The listing builds one solid part. Answer for the finished solid, in the listing's coordinates (mm). A direction names the side the tool comes from. Coordinates: 2 decimals unless noted, no trailing zeros. Loops run counter-clockwise (first coordinate to the right, second up) from the corner with the lowest first, then second, coordinate; pieces in that order, holes last. Notation, with made-up numbers: M 73,-2.5 L 95,-2.5 A29 ccw 95,27.5 Z; hole C 42.5,25 d1. An arc over 180 degrees is marked long. Return JSON: item names as keys, results as strings. Group by question number.
1. Section C-C (x = 83.5) is taken. Write down the section's boundary in (y, z).
2. Which of the six approach directions +Z, -Z, +X, -X, +Y, -Y give full straight-line access (tool end or side, diameter ignored) to faces 4 (the face through (66.5, 0, -6)), 5 (the face through (8, -8, -8)), 6 (the face through (78.189, 10.382, -19.961)), 7 (the face through (19.8, -12.1, -9.2))?
3. Section A-A (x = 47.5) is taken. Write down the section's boundary in (y, z), then the cut area to 3 significant figures.
4. Section B-B (x = 13) is taken. Write down the section's boundary in (y, z).
5. The mould has two halves that part along Z. Classify faces 1 (the face through (94.5, 10, -11.5)), 2 (the face through (80.695, -11.521, -8.834)), 3 (the face through (35.099, -14.985, 0.66)): pulls with the +Z half, pulls with the -Z half, needs draft (parallel to the pull), parting line crosses it, or undercut.
6. Given P1, Ø3, axis at x = 57, y = 6.5, coming from the +Z side; P2, Ø3, axis at x = 60, y = -5, coming from the -Z side; P3, Ø10, axis at x = 50, z = 1, coming from the +Y side, each flat-ended and moving along its own axis, determine where each tip first touches the part or whether it passes through.
7. Straight lines are drawn through the part: L1, parallel to Z at x = 57, y = 0; L2, parallel to Y at x = 67, z = 5; L3, parallel to Z at x = 62.25, y = 0. For each, find the intervals that lie inside material, in ascending order. Write a range as from..to.
```python
from build123d import *


with BuildPart() as part:
    # Sketch1 → Revolve1 (revolve)
    with BuildSketch(Plane.XY):
        with BuildLine():
            Line((44.5, 5.1), (41.555513627, 0))
            Line((41.555513627, 0), (0, 0))
            Line((0, 0), (0, 10))
            Line((0, 10), (1, 11))
            Line((1, 11), (8, 11))
            Line((8, 11), (8, 19))
            Line((8, 19), (16, 19))
            Line((16, 19), (20, 15))
            Line((20, 15), (49.780421209, 15))
            Line((49.780421209, 15), (64.5, 22.5))
            Line((64.5, 22.5), (91.5, 22.5))
            ThreePointArc((91.5, 22.5), (93.621320344, 21.621320344), (94.5, 19.5))
            Line((94.5, 19.5), (94.5, 15))
            Line((94.5, 15), (67.272080403, 14.049180096))
            ThreePointArc((67.272080403, 14.049180096), (66.72452816, 13.805394131), (66.5, 13.249667434))
            Line((66.5, 13.249667434), (66.5, 5.1))
            Line((66.5, 5.1), (44.5, 5.1))
        make_face()
    revolve(axis=Axis((0, 0, 0), (1, 0, 0)))


solid = part.part
```
Worked out:
{
 "1": {"outline": "C 0,0 d45; hole C 0,0 d29.23"},
 "2": {"face 4": "+X", "face 5": "-X", "face 6": "+X, -X", "face 7": "none"},
 "3": {"outline": "C 0,0 d30; hole C 0,0 d10.2", "area": "625 mm^2"},
 "4": {"outline": "C 0,0 d38"},
 "5": {"face 1": "needs draft", "face 2": "undercut", "face 3": "parting line crosses it"},
 "6": {"P1": "z = 18.47", "P2": "z = -20.44", "P3": "y = 17.64"},
 "7": {"L1": "-18.68..-5.1, 5.1..18.68", "L2": "-21.94..-13.07, 13.07..21.94", "L3": "-21.35..-5.1, 5.1..21.35"}
}
